Can you work these out from the model? Positions are in its coordinate system, mm. A direction names the side the tool comes from. Give positions to 0.01 mm unless a question says otherwise; leave off trailing zeros. Loops run counter-clockwise (first coordinate to the right, second up) from the corner with the lowest first, then second, coordinate; pieces in that order, holes last. Notation, with made-up numbers: (86.25, 29.5) -> (143.25, 29.5) arc R18 ccw to (143.25, 63.5) -> close; hole circle Ø11 at (-14.5, 75.25). An arc over 180 degrees is marked (long way). One line per question, with ' | ' between items.
from build123d import *

# Parameters (mm, degrees)
F0_W     = 105.6834086776
F0_H     = 51.6841448843
F0_R     = 17.6030862499
F0_R_2   = 12.5238799036
F0_R_3   = 7.5238607233
F0_R_4   = 3.1994051996
F0_R_5   = 1.8202490714
F1_DEPTH = 4
F2_R     = 17.7598613425
F3_DEPTH = 5
F4_R     = 12.4433858389
F5_DEPTH = 10
F6_R     = 7.5502139522
F7_DEPTH = 15
F8_R     = 3.0929644542
F9_DEPTH = 3


with BuildPart() as f1:
    # F0 (on Front) → F1 (new body)
    with BuildSketch(Plane.XZ):
        Rectangle(F0_W, F0_H)
        Circle(F0_R, mode=Mode.SUBTRACT)
        Circle(F0_R)
        Circle(F0_R_2, mode=Mode.SUBTRACT)
        Circle(F0_R_2)
        Circle(F0_R_3, mode=Mode.SUBTRACT)
        Circle(F0_R_3)
        Circle(F0_R_4, mode=Mode.SUBTRACT)
        Circle(F0_R_4)
        Circle(F0_R_5, mode=Mode.SUBTRACT)
        Circle(F0_R_5)
    extrude(amount=F1_DEPTH)

    # F2 (on face) → F3 (join)
    with BuildSketch(Plane.XZ.offset(4)):
        Circle(F2_R)
    extrude(amount=F3_DEPTH)

    # F4 (on face) → F5 (join)
    with BuildSketch(Plane.XZ.offset(4)):
        Circle(F4_R)
    extrude(amount=F5_DEPTH)

    # F6 (on face) → F7 (join)
    with BuildSketch(Plane.XZ.offset(4)):
        Circle(F6_R)
    extrude(amount=F7_DEPTH)

    # F8 (on Front) → F9 (cut)
    with BuildSketch(Plane.XZ):
        Circle(F8_R)
    extrude(amount=F9_DEPTH, mode=Mode.SUBTRACT)


solid = f1.part
Q1. If we section it at D-D (x = -20): Write out the boundary of the cut face in (y, z).
Entries:
outline: (-4, -25.84) -> (0, -25.84) -> (0, 25.84) -> (-4, 25.84) -> close
Q2. If we section it at B-B (z = 0): Write out the boundary of the cut face in (x, y), plus the area to 3 significant figures.
Entries:
outline: (-52.84, -4) -> (-17.76, -4) -> (-17.76, -9) -> (-12.44, -9) -> (-12.44, -14) -> (-7.55, -14) -> (-7.55, -19) -> (7.55, -19) -> (7.55, -14) -> (12.44, -14) -> (12.44, -9) -> (17.76, -9) -> (17.76, -4) -> (52.84, -4) -> (52.84, 0) -> (3.09, 0) -> (3.09, -3) -> (-3.09, -3) -> (-3.09, 0) -> (-52.84, 0) -> close | area: 782 mm²
Q3. For pin 1 Ø1.5 at (y, z) = (-11.5, -1) entering from -X; pin 2 Ø3.5 at (x, z) = (0, 0) entering from +Y, each with a flat end and sliding along its axis, tell me the tip position at first contact or that it passes through.
Entries:
pin 1: x = -12.44 | pin 2: y = -3
Q4. If we section it at C-C (y = -10): Write out the boundary of the cut face in (x, z).
Entries:
outline: circle Ø24.89 at (0, 0)
Q5. If we section it at A-A (x = 0): Write out the boundary of the cut face in (y, z), plus the area to 3 significant figures.
Entries:
outline: (-19, -7.55) -> (-14, -7.55) -> (-14, -12.44) -> (-9, -12.44) -> (-9, -17.76) -> (-4, -17.76) -> (-4, -25.84) -> (0, -25.84) -> (0, -3.09) -> (-3, -3.09) -> (-3, 3.09) -> (0, 3.09) -> (0, 25.84) -> (-4, 25.84) -> (-4, 17.76) -> (-9, 17.76) -> (-9, 12.44) -> (-14, 12.44) -> (-14, 7.55) -> (-19, 7.55) -> close | area: 566 mm²
Q6. If we mould it in two halves opening along X, with no side actions, what happens to faces 1 (the face through (11.87, -11.46, 3.74)), 2 (the face through (-0.67, -1.48, -3.02)), 3 (the face through (52.842, -2, 0)), 4 (the face through (0, -3, 0))? For each: pulls with the +X half, pulls with the -X half, needs draft (parallel to the pull), parting line crosses it, or undercut.
Entries:
face 1: parting line crosses it | face 2: undercut | face 3: pulls with the +X half | face 4: undercut
Q7. On a 3-axis mill with a long thin cutter (end or side, diameter ignored), from which of +Z, -Z, +X, -X, +Y, -Y can I reach the whole of each face in a straight line? I mean faces 5 (the face through (0, -19, 0)), 6 (the face through (-12, -9, -4)). Say none if no direction works.
Entries:
face 5: +Z, -Z, +X, -X, -Y | face 6: -Y
Q8. If I drill on probe 1 along Z at (x, y) = (0, -1.6); probe 2 along Y at (x, z) = (12, 20.5); probe 3 along Y at (x, z) = (12.5, 11), over which ranges is the centre line in solid material (lowest first)? Write a range as from..to.
Entries:
probe 1: -25.84..-3.09, 3.09..25.84 | probe 2: -4..0 | probe 3: -9..0
